from build123d import *

# Parameters (mm, degrees)
F0_R     = 18.9209145911
F1_DEPTH = 27.178


with BuildPart() as f1:
    # F0 (on Front) → F1 (new body)
    with BuildSketch(Plane.XZ):
        with BuildLine():
            Line((14.8961656121, 60.1436708064), (0, 61.9609303353))
            ThreePointArc((0, 61.9609303353), (-61.9609303353, 0), (0, -61.9609303353))
            Line((0, -61.9609303353), (14.9818155033, -60.1223926024))
            ThreePointArc((14.9818155033, -60.1223926024), (48.8233761364, -38.1501616073), (61.9609303353, 0))
            ThreePointArc((61.9609303353, 0), (48.7961943586, 38.1849224712), (14.8961656121, 60.1436708064))
        make_face()
        with BuildLine():
            ThreePointArc((16.1964445954, -7.1509783156), (0, -17.7048385591), (-16.1964445954, -7.1509783156))
            Line((-16.1964445954, -7.1509783156), (-26.931880042, -7.1509783156))
            Line((-26.931880042, -7.1509783156), (-26.931880042, 7.1509783156))
            Line((-26.931880042, 7.1509783156), (-16.1964445954, 7.1509783156))
            ThreePointArc((-16.1964445954, 7.1509783156), (0, 17.7048385591), (16.1964445954, 7.1509783156))
            Line((16.1964445954, 7.1509783156), (26.931880042, 7.1509783156))
            Line((26.931880042, 7.1509783156), (26.931880042, -7.1509783156))
            Line((26.931880042, -7.1509783156), (16.1964445954, -7.1509783156))
        make_face(mode=Mode.SUBTRACT)
        with BuildLine():
            Line((135.4351173078, 45.4385067882), (14.8961656121, 60.1436708064))
            ThreePointArc((14.8961656121, 60.1436708064), (48.7961943586, 38.1849224712), (61.9609303353, 0))
            ThreePointArc((61.9609303353, 0), (48.8233761364, -38.1501616073), (14.9818155033, -60.1223926024))
            Line((14.9818155033, -60.1223926024), (134.6838830583, -45.4327998856))
            ThreePointArc((134.6838830583, -45.4327998856), (89.9676969368, 0.375627963), (135.4351173078, 45.4385067882))
        make_face()
        with BuildLine():
            ThreePointArc((180.8431782929, 0), (167.5453108139, 32.1191138638), (135.4351173078, 45.4385067882))
            ThreePointArc((135.4351173078, 45.4385067882), (89.9676969368, 0.375627963), (134.6838830583, -45.4327998856))
            ThreePointArc((134.6838830583, -45.4327998856), (167.2786925178, -32.3837144333), (180.8431782929, 0))
        make_face()
        with Locations((135.4046612978, 0)):
            Circle(F0_R, mode=Mode.SUBTRACT)
    extrude(amount=F1_DEPTH)


solid = f1.part
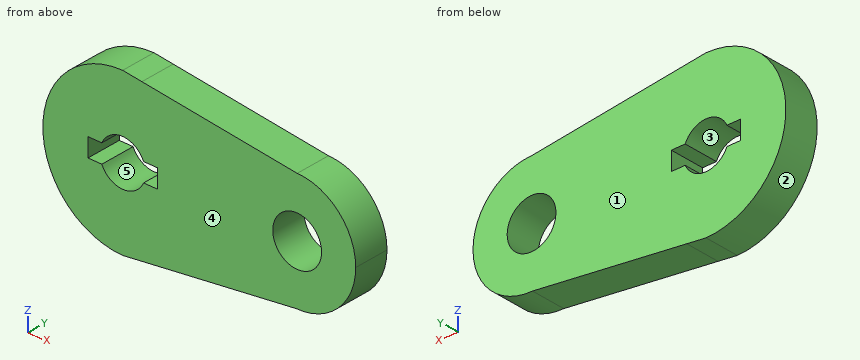
Here's how the part is built. I have some questions about the finished solid (model axes, mm). Face numbers are marked on the shaded views. A direction names the side the tool comes from. Coordinates: 2 decimals unless noted, no trailing zeros. Order: outer loops, then holes, each group sorted by start corner. A loop starts at its lowest first (then second) coordinate and runs counter-clockwise, first axis right, second up. Notation, with made-up numbers: (59.25, 35.5) - (85.25, 35.5) arc R16 ccw to (85.25, 61.5) - close; hole circle Ø2 at (8.5, 24). An arc over 180 degrees is marked (long way). Use CSV: the item, a comma, the result in double quotes. Start each with the question number.
1. Please list where these lines run through material, in increasing order: line 1 (Z direction, x = -13, y = -24); line 2 (Z direction, x = 15, y = -10.5); line 3 (Z direction, x = 90.5, y = -12.25). Write a range as from..to.
2. If we mould it in two halves opening along Z, with no side actions, what happens to the marked faces 1, 2 and 3? For each: +Z half, -Z half, draft (parallel to the pull), parting line (faces both ways), or undercut.
3. Suppose I cut it at A-A on y = -21.25. List the corners of the cut face in (x, z) for me, then the cut area to 3 significant figures.
4. Suppose I cut it at C-C on x = 72. List the corners of the cut face in (y, z) for me, then the cut area to 3 significant figures.
5. For the marked faces 4 and 5, which set-ups out of +Z, -Z, +X, -X, +Y, -Y let a thin tool reach every point of the face, with its end or its side?
6. I'm going to push flat-ended pins straight in: pin 1 (5 mm diameter, centred on y = -3, z = -22.5, fed in from +X); pin 2 (8 mm diameter, centred on x = 68.5, z = 45, fed in from +Y); pin 3 (1 mm diameter, centred on y = -18.5, z = 35, fed in from +X); pin 4 (10 mm diameter, centred on y = -7, z = -17, fed in from +X). Where does each tip first touch, or does it pass through?
7. Suppose I cut it at B-B on z = 34.5. List the corners of the cut face in (x, y) for me.
Output:
1,line 1,"z = -60.58..-12.02, 12.02..60.58"
1,line 2,"z = -60.12..-9.41, 9.41..60.13"
1,line 3,"z = -50.85..50.92"
2,face 1,"draft"
2,face 2,"parting line"
2,face 3,"undercut"
3,outline,"(0, -61.96) - (134.68, -45.43) arc R45.44 ccw (long way) to (135.44, 45.44) - (0, 61.96) arc R61.96 ccw to start; hole (-26.93, -7.15) - (-16.2, -7.15) arc R17.7 ccw to (16.2, -7.15) - (26.93, -7.15) - (26.93, 7.15) - (16.2, 7.15) arc R17.7 ccw to (-16.2, 7.15) - (-26.93, 7.15) - close; hole circle Ø37.84 at (135.4, 0)"
3,area,"21,400 mm2"
4,outline,"(-27.18, -53.13) - (0, -53.13) - (0, 53.18) - (-27.18, 53.18) - close"
4,area,"2,890 mm2"
5,face 4,"+Z, -Z, +X, -X, -Y"
5,face 5,"+Y, -Y"
6,pin 1,"stops at x = 176.2"
6,pin 2,"stops at y = 0"
6,pin 3,"stops at x = 164.98"
6,pin 4,"stops at x = 179.23"
7,outline,"(-51.47, -27.18) - (164.98, -27.18) - (164.98, 0) - (-51.47, 0) - close"
